Geometry: final body of the model. Coordinates: model frame, mm. A direction names the side the tool comes from. Coordinates: 2 decimals unless noted, no trailing zeros. Order: outer loops, then holes, each group sorted by start corner. A loop starts at its lowest first (then second) coordinate and runs counter-clockwise, first axis right, second up. Notation, with made-up numbers: M 27.25,21.25 L 73.25,21.25 A15 cw 73.25,30.25 Z; hole C 50.25,1.25 d4. An arc over 180 degrees is marked long. Write item = value, one per line.
from build123d import *

# Parameters (mm, degrees)
F1_DEPTH  = 69.85
F2_W      = 3.175
F2_H      = 6.35
F3_DEPTH  = 40.005
F4_SIZE   = 0.508
F5_R      = 1.5875
F6_DEPTH  = 1.651
F7_R      = 1.5875
F8_DEPTH  = 1.651
F9_W      = 30.2895
F9_H      = 4.2418
F10_DEPTH = 27.94
F11_R     = 3.81
F12_DEPTH = 1.651
F14_DEPTH = 30.2905
F16_DEPTH = 2.54


with BuildPart() as f1:
    # F0 (on Top) → F1 (new body)
    with BuildSketch(Plane.XY):
        with BuildLine():
            Line((2.54, 40.005), (-6.985, 40.005))
            Line((-6.985, 40.005), (-6.985, 10.16))
            ThreePointArc((-6.985, 10.16), (-8.8448719395, 5.6698719395), (-13.335, 3.81))
            Line((-13.335, 3.81), (-26.67, 3.81))
            ThreePointArc((-26.67, 3.81), (-30.2895, 0.1905), (-26.67, -3.429))
            Line((-26.67, -3.429), (-17.78, -3.429))
            ThreePointArc((-17.78, -3.429), (-16.51, -2.159), (-17.78, -0.889))
            Line((-17.78, -0.889), (-25.4, -0.889))
            Line((-25.4, -0.889), (-25.4, 0))
            Line((-25.4, 0), (0, 0))
            Line((0, 0), (0, -3.175))
            Line((0, -3.175), (1.2192, -3.175))
            ThreePointArc((1.2192, -3.175), (2.1531466366, -2.7881466366), (2.54, -1.8542))
            Line((2.54, -1.8542), (2.54, 40.005))
        make_face()
    extrude(amount=F1_DEPTH)

    # F2 (on face) → F3 (join, through all)
    with BuildSketch(Plane(origin=(0, 40.005, 0), x_dir=(-1, 0, 0), z_dir=(0, 1, 0))):
        with Locations((2.2225, 73.025)):
            Rectangle(F2_W, F2_H)
    extrude(amount=-F3_DEPTH)

    # F4
    f4_edges = [f1.edges().sort_by_distance(p)[0] for p in [
        (-0.635, 20.0025, 76.2),
        (-3.81, 20.0025, 76.2),
    ]]
    chamfer(f4_edges, length=F4_SIZE)

    # F5 (on face) → F6 (cut)
    with BuildSketch(Plane(origin=(0, 40.005, 0), x_dir=(-1, 0, 0), z_dir=(0, 1, 0))):
        with Locations((2.2225, 6.35)):
            Circle(F5_R)
        with Locations((2.2225, 31.75)):
            Circle(F5_R)
        with Locations((2.2225, 57.15)):
            Circle(F5_R)
    extrude(amount=-F6_DEPTH, mode=Mode.SUBTRACT)

    # F7 (on face) → F8 (cut)
    with BuildSketch(Plane.XZ):
        with Locations((-2.2225, 57.15)):
            Circle(F7_R)
        with Locations((-2.2225, 38.1)):
            Circle(F7_R)
    extrude(amount=-F8_DEPTH, mode=Mode.SUBTRACT)

    # F9 (on face) → F10 (cut)
    with BuildSketch(Plane(origin=(0, 0, 0), x_dir=(1, 0, 0), z_dir=(0, 0, -1))):
        with Locations((-15.14475, 1.3081)):
            Rectangle(F9_W, F9_H)
    extrude(amount=-F10_DEPTH, mode=Mode.SUBTRACT)

    # F11 (on face) → F12 (cut)
    with BuildSketch(Plane.XZ.offset(-0.8128)):
        with Locations((-6.985, 22.098)):
            Circle(F11_R)
        with Locations((-19.558, 11.938)):
            Circle(F11_R)
    extrude(amount=-F12_DEPTH, mode=Mode.SUBTRACT)

    # F13 (on face) → F14 (cut, through all)
    with BuildSketch(Plane(origin=(0, 0, 0), x_dir=(0, -1, 0), z_dir=(-1, 0, 0))):
        Polygon((3.429, 32.1818), (-0.8128, 27.94), (3.429, 27.94), align=None)
    extrude(amount=F14_DEPTH, mode=Mode.SUBTRACT)

    # F15 (on face) → F16 (cut, through all)
    with BuildSketch(Plane.XZ.offset(3.429)):
        Polygon((-12.7, 42.3418), (-25.4, 29.6418), (-12.7, 29.6418), align=None)
    extrude(amount=-F16_DEPTH, mode=Mode.SUBTRACT)


solid = f1.part
1) Set-up query: faces 5 (the face through (-6.985, 25, 34)), 6 (the face through (-22, -0.889, 49)), 7 (the face through (-3.81, 20, 73)). Return all of +Z, -Z, +X, -X, +Y, -Y with unobstructed straight access to the full face (end or side cutting, diameter ignored); none if empty.
Numbers:
face_5 = +Z, -Z, -X, +Y
face_6 = +Z, -Z
face_7 = +Z, -X, +Y, -Y
2) Section D-D, the plane x = -8.5. Return loops of the section in (y, z).
Numbers:
outline = M 0,28.75 L 0.81,27.94 L 0.81,25.59 L 2.46,25.59 L 2.46,18.6 L 0.81,18.6 L 0.81,0 L 6.04,0 L 6.04,69.85 L 0,69.85 Z
3) Mould query, pull axis Z, two halves, no side actions, for faces 1 (the face through (-2, 20, 76.2)), 2 (the face through (-16.51, -2.19, 53.33)), 3 (the face through (-2.57, 0.81, 55.6)), 4 (the face through (-20.89, -2.18, 34.15)). Classes: pulls with the +Z half, pulls with the -Z half, needs draft (parallel to the pull), parting line crosses it, or undercut.
Numbers:
face_1 = pulls with the +Z half
face_2 = needs draft
face_3 = undercut
face_4 = pulls with the -Z half
4) Section C-C, the plane y = 13.5. Return loops of the section in (x, z) (3 decimals), and give its area (3 significant figures).
Numbers:
outline = M -6.985,0 L 2.54,0 L 2.54,69.85 L -0.635,69.85 L -0.635,75.692 L -1.143,76.2 L -3.302,76.2 L -3.81,75.692 L -3.81,69.85 L -6.985,69.85 Z
area = 685 mm²
5) Line query: L1, parallel to Y at x = -21, z = 57; L2, parallel to X at y = 22.5, z = 68 (3 decimals); L3, parallel to Z at x = 1.5, y = 1.5. Output: solid intervals per line, ascending.
Numbers:
L1 = -3.43 to -0.89, 0 to 3.81
L2 = -6.985 to 2.54
L3 = 0 to 69.85
6) Section B-B, the plane x = -22. Return loops of the section in (y, z).
Numbers:
outline = M -3.43,33.04 L -0.89,33.04 L -0.89,69.85 L -3.43,69.85 Z; M 0,28.75 L 0.81,27.94 L 0.81,14.86 L 2.46,14.86 L 2.46,9.01 L 0.81,9.01 L 0.81,0 L 3.81,0 L 3.81,69.85 L 0,69.85 Z
7) Pin query (flat end, axial travel): pin 1 (6 mm diameter, centred on x = -20.5, z = 52.5, fed in from +Y); pin 2 (6 mm diameter, centred on y = 31.5, z = 46, fed in from -X) (3 decimals); pin 3 (10 mm diameter, centred on x = -6.985, z = 22.098, fed in from -Y); pin 4 (3.5 mm diameter, centred on x = -2.5, z = 57.5, fed in from +Y) (3 decimals). Return the tip coordinate at first contact, or that it passes through.
Numbers:
pin_1 = 3.81
pin_2 = -6.985
pin_3 = 0.81
pin_4 = 40.005
